```python
from build123d import *

# Parameters (mm, degrees)
F0_R     = 19.05
F1_DEPTH = 50.8
F0_R_2   = 9.525
F2_DEPTH = 19.05


with BuildPart() as f1:
    # F0 (on Front) → F1 (new body)
    with BuildSketch(Plane.XZ):
        with BuildLine():
            ThreePointArc((29.099356, -12.7), (31.080275, -6.486831), (31.75, 0))
            ThreePointArc((31.75, 0), (31.080275, 6.486831), (29.099356, 12.7))
            ThreePointArc((29.099356, 12.7), (0, 31.75), (-29.099356, 12.7))
            ThreePointArc((-29.099356, 12.7), (-31.75, 0), (-29.099356, -12.7))
            ThreePointArc((-29.099356, -12.7), (0, -31.75), (29.099356, -12.7))
        make_face()
        Circle(F0_R, mode=Mode.SUBTRACT)
    extrude(amount=F1_DEPTH)

    # F0 (on Front) → F2 (join)
    with BuildSketch(Plane.XZ):
        with BuildLine():
            ThreePointArc((-29.099356, -12.7), (-31.75, 0), (-29.099356, 12.7))
            Line((-29.099356, 12.7), (-52.149535, 12.7))
            ThreePointArc((-52.149535, 12.7), (-64.849535, 0), (-52.149535, -12.7))
            Line((-52.149535, -12.7), (-29.099356, -12.7))
        make_face()
        with Locations((-52.149535, 0)):
            Circle(F0_R_2, mode=Mode.SUBTRACT)
        with BuildLine():
            ThreePointArc((29.099356, 12.7), (31.080275, 6.486831), (31.75, 0))
            ThreePointArc((31.75, 0), (31.080275, -6.486831), (29.099356, -12.7))
            Line((29.099356, -12.7), (72.10981, -12.7))
            ThreePointArc((72.10981, -12.7), (84.80981, 0), (72.10981, 12.7))
            Line((72.10981, 12.7), (29.099356, 12.7))
        make_face()
        with BuildLine():
            ThreePointArc((72.10981, 9.525), (81.63481, 0), (72.10981, -9.525))
            Line((72.10981, -9.525), (44.16981, -9.525))
            ThreePointArc((44.16981, -9.525), (34.64481, 0), (44.16981, 9.525))
            Line((44.16981, 9.525), (72.10981, 9.525))
        make_face(mode=Mode.SUBTRACT)
    extrude(amount=F2_DEPTH)


solid = f1.part
```
Geometry check sheet. Reference: the model listing, model coordinates, mm. A direction names the side the tool comes from. Round coordinates to 2 decimals unless told otherwise and drop trailing zeros. Order: outer loops, then holes, each group sorted by start corner. A loop starts at its lowest first (then second) coordinate and runs counter-clockwise, first axis right, second up. Notation, with made-up numbers: (-16.5, 31.5) - (13.5, 31.5) arc R21 cw to (13.5, 61.5) - close; hole circle Ø6 at (7.5, 46.5). An arc over 180 degrees is marked (long way). Use a Markdown table: item, result. Add a question column.
1) Section check C-C (y = -42). Record the cut outline in (x, z).
2) Section check D-D (z = 5.5). Record the cut outline in (x, y).
3) Thickness scan on line 1 along Z through (x, y) = (55, -9) (3 decimals); line 2 along X through (y, z) = (-9, -4.5); line 3 along X through (y, z) = (-30, -1). Record the ranges inside material, lowest first.
4) Gauge pin test, flat ends, axial feed: P1, Ø20.5, axis at x = 49, z = 6.5, coming from the -Y side; P2, Ø1.5, axis at x = 46, z = -8.5, coming from the -Y side; P3, Ø8, axis at y = -5.5, z = -10, coming from the +X side; P4, Ø6, axis at x = 33, y = -15, coming from the +Z side. Record the tip position at first contact, or that the pin passes through.
5) Section check B-B (x = 0). Record the cut outline in (y, z), then the cut area to 3 significant figures.
6) Set-up check for faces 4 (the cylindrical face through (84.807, -9.392, -0.279)), 5 (the flat face through (15, 0, -12)), 6 (the cylindrical face through (81.633, -9.392, 0.209)), 7 (the flat face through (51, -9, 12.7)), 8 (the flat face through (50, -9, -12.7)): record each of +Z, -Z, +X, -X, +Y, -Y from which the full face is reachable in a straight line by a thin tool's end or side.
7) Section check A-A (y = -2.5). Record the cut outline in (x, z) (3 decimals).
8) Mould release check, pull along Z, two halves, no side actions. Record for faces 1 (the cylindrical face through (34.647, -9.392, -0.209)), 2 (the flat face through (-40, -9, 12.7)), 3 (the flat face through (-41, -9, -12.7)): released by +Z, released by -Z, zero draft, split by the parting line, or undercut.
Established:
| question | item | result |
|---|---|---|
| 1 | outline | (-29.1, -12.7) arc R31.75 ccw to (29.1, -12.7) arc R31.75 ccw to (31.75, 0) arc R31.75 ccw to (29.1, 12.7) arc R31.75 ccw to (-29.1, 12.7) arc R31.75 ccw to start; hole circle Ø38.1 at (0, 0) |
| 2 | outline | (-63.6, -19.05) - (-59.93, -19.05) - (-59.93, 0) - (-63.6, 0) - close; (-44.37, -19.05) - (-31.27, -19.05) - (-31.27, -50.8) - (-18.24, -50.8) - (-18.24, 0) - (-44.37, 0) - close; (18.24, -50.8) - (31.27, -50.8) - (31.27, -19.05) - (36.39, -19.05) - (36.39, 0) - (18.24, 0) - close; (79.89, -19.05) - (83.56, -19.05) - (83.56, 0) - (79.89, 0) - close |
| 3 | line 1 | -12.7 to -9.525, 9.525 to 12.7 |
| 3 | line 2 | -64.03 to -60.54, -43.75 to -18.51, 18.51 to 35.77, 80.5 to 83.99 |
| 3 | line 3 | -31.73 to -19.02, 19.02 to 31.73 |
| 4 | P1 | y = -19.05 |
| 4 | P2 | through |
| 4 | P3 | x = 83.3 |
| 4 | P4 | z = 12.7 |
| 5 | outline | (-50.8, -31.75) - (0, -31.75) - (0, -19.05) - (-50.8, -19.05) - close; (-50.8, 19.05) - (0, 19.05) - (0, 31.75) - (-50.8, 31.75) - close |
| 5 | area | 1,290 mm2 |
| 6 | face 4 | +X, +Y, -Y |
| 6 | face 5 | +Z, -Z, +X, -X, +Y |
| 6 | face 6 | +Y, -Y |
| 6 | face 7 | +Z, +X, +Y, -Y |
| 6 | face 8 | -Z, +X, +Y, -Y |
| 7 | outline | (-52.15, -12.7) - (-29.099, -12.7) arc R31.75 ccw to (29.099, -12.7) - (72.11, -12.7) arc R12.7 ccw to (72.11, 12.7) - (29.099, 12.7) arc R31.75 ccw to (-29.099, 12.7) - (-52.15, 12.7) arc R12.7 ccw to start; hole circle Ø19.05 at (-52.15, 0); hole circle Ø38.1 at (0, 0); hole (44.17, -9.525) - (72.11, -9.525) arc R9.525 ccw to (72.11, 9.525) - (44.17, 9.525) arc R9.525 ccw to start |
| 8 | face 1 | undercut |
| 8 | face 2 | released by +Z |
| 8 | face 3 | released by -Z |
